from build123d import *

# Parameters (mm, degrees)
SALIENTE_EXTRUIR1_DEPTH = 1
CROQUIS2_W              = 6
CROQUIS2_H              = 6
CROQUIS2_R              = 1.75
SALIENTE_EXTRUIR2_DEPTH = 8.5
CROQUIS3_W              = 4.14
CROQUIS3_H              = 6
SALIENTE_EXTRUIR3_DEPTH = 1


with BuildPart() as part:
    # Croquis1 → Saliente-Extruir1 (new body)
    with BuildSketch(Plane(origin=(0, 0, 0), x_dir=(1, 0, 0), z_dir=(0, 1, 0))):
        Polygon((0, 0), (0, -101.83), (6.27, -101.83), (38.16, -70.885), (45.4, -70.885), (45.4, -30.945), (38.16, -30.945), (6.27, 0), align=None)
    extrude(amount=SALIENTE_EXTRUIR1_DEPTH)

    # Croquis2 → Saliente-Extruir2 (add)
    # profile 1 of 3: a face of its own
    with BuildSketch(Plane(origin=(0, 1, 0), x_dir=(1, 0, 0), z_dir=(0, 1, 0))):
        with Locations((14.54, -27.515)):
            Rectangle(CROQUIS2_W, CROQUIS2_H)
        with Locations(Location((14.54, -27.515, 0), (0, 0, 270))):
            Circle(CROQUIS2_R, mode=Mode.SUBTRACT)
    # profile 2 of 3: a face of its own
    with BuildSketch(Plane(origin=(0, 1, 0), x_dir=(1, 0, 0), z_dir=(0, 1, 0))):
        with Locations((14.54, -74.315)):
            Rectangle(CROQUIS2_W, CROQUIS2_H)
        with Locations(Location((14.54, -74.315, 0), (0, 0, 270))):
            Circle(CROQUIS2_R, mode=Mode.SUBTRACT)
    # profile 3 of 3: a face of its own
    with BuildSketch(Plane(origin=(0, 1, 0), x_dir=(1, 0, 0), z_dir=(0, 1, 0))):
        with Locations((46.54, -50.915)):
            Rectangle(CROQUIS2_W, CROQUIS2_H)
        with Locations(Location((46.54, -50.915, 0), (0, 0, 130.649396827))):
            Circle(CROQUIS2_R, mode=Mode.SUBTRACT)
    extrude(amount=SALIENTE_EXTRUIR2_DEPTH)

    # Croquis3 → Saliente-Extruir3 (add)
    with BuildSketch(Plane.XZ.offset(-1)):
        with Locations((47.47, 50.915)):
            Rectangle(CROQUIS3_W, CROQUIS3_H)
    extrude(amount=SALIENTE_EXTRUIR3_DEPTH)


solid = part.part
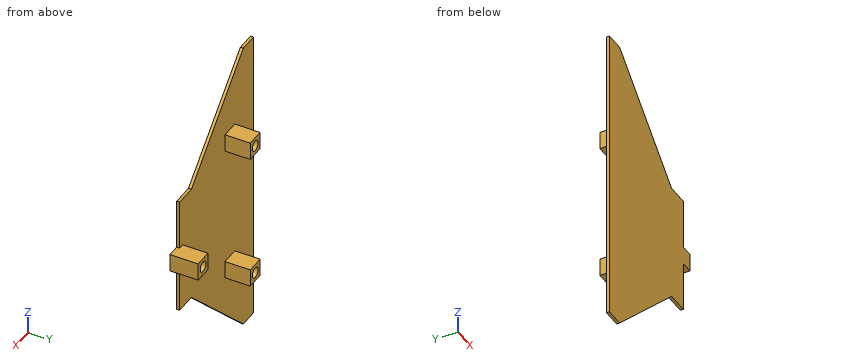
Check sheet for the modelled part. Datum: model origin and axes. Units: mm. Give positions to 0.01 mm unless a question says otherwise; leave off trailing zeros. Order: outer loops, then holes, each group sorted by start corner. A loop starts at its lowest first (then second) coordinate and runs counter-clockwise, first axis right, second up. Notation, with made-up numbers: (56, 1) - (82, 1) arc R24 cw to (82, 18) - close; hole circle Ø6 at (23, 26). An arc over 180 degrees is marked (long way). Answer as CSV lines item,"result".
1. Section check C-C (z = 73.5). Record the boundary of the cut face in (x, y).
Result sheet:
outline,"(0, 0) - (35.47, 0) - (35.47, 1) - (17.54, 1) - (17.54, 9.5) - (16.09, 9.5) - (16.09, 1) - (12.99, 1) - (12.99, 9.5) - (11.54, 9.5) - (11.54, 1) - (0, 1) - close"
2. Section check B-B (x = 46.54). Record the boundary of the cut face in (y, z) (3 decimals).
Result sheet:
outline,"(0, 47.915) - (9.5, 47.915) - (9.5, 49.165) - (1, 49.165) - (1, 52.665) - (9.5, 52.665) - (9.5, 53.915) - (0, 53.915) - close"
3. Go/stop test with flat-tipped pins: P1, Ø12, axis at x = 28, z = 74.5, coming from the -Y side; P2, Ø5, axis at x = 15.5, y = 5.5, coming from the -Z side (3 decimals); P3, Ø0.5, axis at y = 0.5, z = 37, coming from the +X side; P4, Ø1.8, axis at y = 4, z = 28.5, coming from the +X side. Record where each tip stops, or that it passes through.
Result sheet:
P1,"y = 0"
P2,"z = 24.515"
P3,"x = 45.4"
P4,"x = 17.54"
4. Section check A-A (y = 3.75). Record the boundary of the cut face in (x, z) (3 decimals).
Result sheet:
outline,"(11.54, 24.515) - (17.54, 24.515) - (17.54, 30.515) - (11.54, 30.515) - close; (11.54, 71.315) - (17.54, 71.315) - (17.54, 77.315) - (11.54, 77.315) - close; (43.54, 47.915) - (49.54, 47.915) - (49.54, 53.915) - (43.54, 53.915) - close; hole circle Ø3.5 at (14.54, 27.515); hole circle Ø3.5 at (14.54, 74.315); hole circle Ø3.5 at (46.54, 50.915)"
5. Scan lines: probe 1 along X at (y, z) = (1.75, 74.5); probe 2 along Z at (x, y) = (46.54, 7.25) (3 decimals); probe 3 along Z at (x, y) = (15.5, 8) (3 decimals). Record each from-to range of solid material in increasing order. Write a range as from..to.
Result sheet:
probe 1,"11.54..12.8, 16.28..17.54"
probe 2,"47.915..49.165, 52.665..53.915"
probe 3,"24.515..26.052, 28.978..30.515, 71.315..72.852, 75.778..77.315"
6. Section check D-D (x = 14.54). Record the boundary of the cut face in (y, z) (3 decimals).
Result sheet:
outline,"(0, 8.025) - (1, 8.025) - (1, 24.515) - (9.5, 24.515) - (9.5, 25.765) - (1, 25.765) - (1, 29.265) - (9.5, 29.265) - (9.5, 30.515) - (1, 30.515) - (1, 71.315) - (9.5, 71.315) - (9.5, 72.565) - (1, 72.565) - (1, 76.065) - (9.5, 76.065) - (9.5, 77.315) - (1, 77.315) - (1, 93.805) - (0, 93.805) - close"
